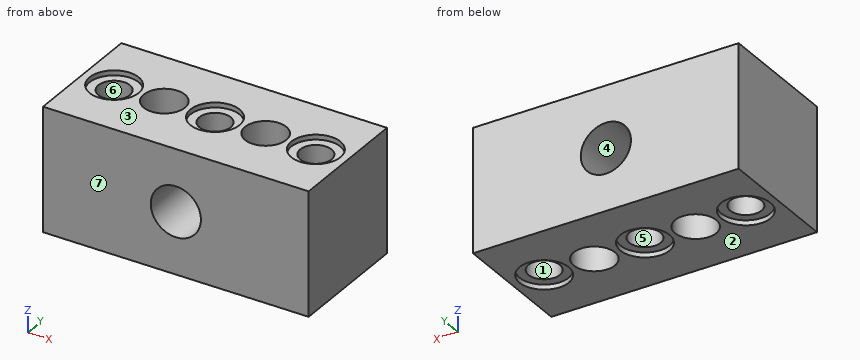
```python
from build123d import *

# Parameters (mm, degrees)
BOSS_EXTRUDE1_DEPTH      = 12.55
BOSS_EXTRUDE1_DEPTH_BACK = 12.55
SKETCH1_W                = 54
SKETCH1_H                = 25.4
CUT_EXTRUDE1_REACH       = 41.136
SKETCH3_R                = 5.1
SKETCH5_R                = 5
CUT_EXTRUDE2_DEPTH       = 1
SKETCH6_R                = 3.2
CUT_EXTRUDE3_DEPTH       = 4.6
CUT_EXTRUDE4_REACH       = 37.645
SKETCH7_R                = 2
CUT_EXTRUDE5_REACH       = 40.991
SKETCH8_R                = 4.2
SKETCH9_R                = 5
CUT_EXTRUDE6_DEPTH       = 1
SKETCH10_R               = 3.2
CUT_EXTRUDE7_DEPTH       = 4.6
SKETCH11_R               = 2
CUT_EXTRUDE8_DEPTH       = 36.64463494


with BuildPart() as part:
    # Sketch1 → Boss-Extrude1 (new, two sides: drawn at the far end of the back side and taken through both)
    with BuildSketch(Plane.XY.offset(-BOSS_EXTRUDE1_DEPTH_BACK)):
        Rectangle(SKETCH1_W, SKETCH1_H)
    extrude(amount=BOSS_EXTRUDE1_DEPTH + BOSS_EXTRUDE1_DEPTH_BACK)

    # Sketch3 → Cut-Extrude1 (cut, up to next)
    with BuildSketch(Plane.XZ.offset(12.7), mode=Mode.PRIVATE) as cut_extrude1_sk1:
        Circle(SKETCH3_R)
    cut_extrude1_tool1 = extrude(cut_extrude1_sk1.sketch, amount=-CUT_EXTRUDE1_REACH, mode=Mode.PRIVATE) & part.part
    add(cut_extrude1_tool1.solids().sort_by_distance((0, -12.7, 0))[0], mode=Mode.SUBTRACT)

    # Sketch5 → Cut-Extrude2 (cut)
    with BuildSketch(Plane.XY.offset(12.55)):
        with Locations((20.5, 0)):
            Circle(SKETCH5_R)
        with Locations(Location((-20.5, 0, 0), (0, 0, 180))):
            Circle(SKETCH5_R)
    cut_extrude2 = extrude(amount=-CUT_EXTRUDE2_DEPTH, mode=Mode.SUBTRACT)

    # Sketch6 → Cut-Extrude3 (cut)
    with BuildSketch(Plane.XY.offset(11.55)):
        with Locations((20.5, 0)):
            Circle(SKETCH6_R)
        with Locations(Location((-20.5, 0, 0), (0, 0, 180))):
            Circle(SKETCH6_R)
    cut_extrude3 = extrude(amount=-CUT_EXTRUDE3_DEPTH, mode=Mode.SUBTRACT)

    # Sketch7 → Cut-Extrude4 (cut, up to next)
    with BuildSketch(Plane.XY.offset(6.95), mode=Mode.PRIVATE) as cut_extrude4_sk1:
        with Locations((20.5, 0)):
            Circle(SKETCH7_R)
    cut_extrude4_tool1 = extrude(cut_extrude4_sk1.sketch, amount=-CUT_EXTRUDE4_REACH, mode=Mode.PRIVATE) & part.part
    # Sketch7 → Cut-Extrude4 (cut, up to next)
    with BuildSketch(Plane.XY.offset(6.95), mode=Mode.PRIVATE) as cut_extrude4_sk2:
        with Locations(Location((-20.5, 0, 0), (0, 0, 180))):
            Circle(SKETCH7_R)
    cut_extrude4_tool2 = extrude(cut_extrude4_sk2.sketch, amount=-CUT_EXTRUDE4_REACH, mode=Mode.PRIVATE) & part.part
    add(cut_extrude4_tool1.solids().sort_by_distance((20.5, 0, 6.95))[0], mode=Mode.SUBTRACT)
    add(cut_extrude4_tool2.solids().sort_by_distance((-20.5, 0, 6.95))[0], mode=Mode.SUBTRACT)

    # Mirror1: Cut-Extrude2 across plane
    add(cut_extrude2.mirror(Plane.XY), mode=Mode.SUBTRACT)

    # Mirror2: Cut-Extrude3 across plane
    add(cut_extrude3.mirror(Plane.XY), mode=Mode.SUBTRACT)

    # Sketch8 → Cut-Extrude5 (cut, up to next)
    with BuildSketch(Plane.XY.offset(12.55), mode=Mode.PRIVATE) as cut_extrude5_sk1:
        with Locations((10.3, 0)):
            Circle(SKETCH8_R)
    cut_extrude5_tool1 = extrude(cut_extrude5_sk1.sketch, amount=-CUT_EXTRUDE5_REACH, mode=Mode.PRIVATE) & part.part
    # Sketch8 → Cut-Extrude5 (cut, up to next)
    with BuildSketch(Plane.XY.offset(12.55), mode=Mode.PRIVATE) as cut_extrude5_sk2:
        with Locations(Location((-10.3, 0, 0), (0, 0, 180))):
            Circle(SKETCH8_R)
    cut_extrude5_tool2 = extrude(cut_extrude5_sk2.sketch, amount=-CUT_EXTRUDE5_REACH, mode=Mode.PRIVATE) & part.part
    add(cut_extrude5_tool1.solids().sort_by_distance((10.3, 0, 12.55))[0], mode=Mode.SUBTRACT)
    add(cut_extrude5_tool2.solids().sort_by_distance((-10.3, 0, 12.55))[0], mode=Mode.SUBTRACT)

    # Sketch9 → Cut-Extrude6 (cut)
    with BuildSketch(Plane.XY.offset(12.55)):
        Circle(SKETCH9_R)
    cut_extrude6 = extrude(amount=-CUT_EXTRUDE6_DEPTH, mode=Mode.SUBTRACT)

    # Sketch10 → Cut-Extrude7 (cut)
    with BuildSketch(Plane.XY.offset(11.55)):
        Circle(SKETCH10_R)
    cut_extrude7 = extrude(amount=-CUT_EXTRUDE7_DEPTH, mode=Mode.SUBTRACT)

    # Sketch11 → Cut-Extrude8 (cut, through all)
    with BuildSketch(Plane.XY.offset(6.95)):
        Circle(SKETCH11_R)
    extrude(amount=-CUT_EXTRUDE8_DEPTH, mode=Mode.SUBTRACT)

    # Mirror3: Cut-Extrude6, Cut-Extrude7 across plane
    add(cut_extrude6.mirror(Plane.XY), mode=Mode.SUBTRACT)
    add(cut_extrude7.mirror(Plane.XY), mode=Mode.SUBTRACT)


solid = part.part
```
The model under review builds one solid part; all positions refer to its coordinate system, in mm. Face numbers are marked on the shaded views. A direction names the side the tool comes from. Round coordinates to 2 decimals unless told otherwise and drop trailing zeros. Loops run counter-clockwise (first coordinate to the right, second up) from the corner with the lowest first, then second, coordinate; pieces in that order, holes last.
Item 1: Take a section at C-C (x = 20.5). Write out the cut boundary in (y, z).
Determined:
outline: (-12.7, -12.55) - (-5, -12.55) - (-5, -11.55) - (-3.2, -11.55) - (-3.2, -6.95) - (-2, -6.95) - (-2, 6.95) - (-3.2, 6.95) - (-3.2, 11.55) - (-5, 11.55) - (-5, 12.55) - (-12.7, 12.55) - close; (2, -6.95) - (3.2, -6.95) - (3.2, -11.55) - (5, -11.55) - (5, -12.55) - (12.7, -12.55) - (12.7, 12.55) - (5, 12.55) - (5, 11.55) - (3.2, 11.55) - (3.2, 6.95) - (2, 6.95) - close
Item 2: For line 1 (Y direction, x = 20.5, z = 11.9); line 2 (X direction, y = -0.75, z = 6.5); line 3 (Z direction, x = 1, y = 4), list the stretches that pass through material, from the lowest coordinate up.
Determined:
line 1: y = -12.7 to -5, 5 to 12.7
line 2: x = -27 to -22.35, -18.65 to -14.43, -6.17 to -1.85, 1.85 to 6.17, 14.43 to 18.65, 22.35 to 27
line 3: z = -11.55 to -5, 5 to 11.55
Item 3: Mouldability with a two-part tool opening along Z and no side actions: class the marked faces 1, 2, 3 and 4 as released by +Z, released by -Z, zero draft, split by the parting line, or undercut.
Determined:
face 1: zero draft
face 2: released by -Z
face 3: released by +Z
face 4: undercut
Item 4: Take a section at D-D (z = -7.5). Write out the cut boundary in (x, y), then the cut area to 3 significant figures.
Determined:
outline: (-27, -12.7) - (27, -12.7) - (27, 12.7) - (-27, 12.7) - close; hole circle Ø6.4 at (-20.5, 0); hole circle Ø8.4 at (-10.3, 0); hole circle Ø6.4 at (0, 0); hole circle Ø8.4 at (10.3, 0); hole circle Ø6.4 at (20.5, 0)
area: 1,160 mm2
Item 5: Take a section at B-B (z = 0). Write out the cut boundary in (x, y), then the cut area to 3 significant figures.
Determined:
outline: (-27, -12.7) - (-5.1, -12.7) - (-5.1, 12.7) - (-27, 12.7) - close; (5.1, -12.7) - (27, -12.7) - (27, 12.7) - (5.1, 12.7) - close; hole circle Ø4 at (-20.5, 0); hole circle Ø8.4 at (-10.3, 0); hole circle Ø8.4 at (10.3, 0); hole circle Ø4 at (20.5, 0)
area: 977 mm2
Item 6: For the marked faces 5, 6 and 7, list the 3-axis set-ups (+Z, -Z, +X, -X, +Y, -Y) from which the entire face can be reached by the end or side of a thin tool; tool diameter is ignored.
Determined:
face 5: -Z
face 6: +Z
face 7: +Z, -Z, +X, -X, -Y
Item 7: Clearance check with flat-ended pins moving along their axes: pin 1 Ø2.5 at (x, y) = (0, 0) entering from +Z; pin 2 Ø3 at (x, y) = (20, -2.5) entering from -Z; pin 3 Ø5 at (x, y) = (-20.5, 0) entering from +Z; pin 4 Ø1.5 at (x, y) = (-19.5, 4) entering from +Z. State where each tip first meets the part, or that it passes through.
Determined:
pin 1: passes through
pin 2: stops at z = -11.55
pin 3: stops at z = 6.95
pin 4: stops at z = 11.55
Item 8: Take a section at A-A (x = 0). Give the number of separate pieces and of enclosed holes in the cut face, then the cut area to 3 significant figures.
Determined:
separate pieces: 4
enclosed holes: 0
area: 285 mm2
